Here's how the part is built. I have some questions about the finished solid (model axes, mm). A direction names the side the tool comes from. Coordinates: 2 decimals unless noted, no trailing zeros. Write each loop counter-clockwise with the first axis right and the second up, starting at its lowest first coordinate (ties: lowest second). Pieces come first, ordered by that corner, then holes.
(1) For pin 1 Ø12 at (x, y) = (18.5, -2.5) entering from -Z; pin 2 Ø12 at (y, z) = (-14.5, -13.5) entering from +X; pin 3 Ø1 at (x, y) = (92, 4) entering from +Z, each with a flat end and sliding along its axis, tell me the tip position at first contact or that it passes through.
(2) Please list where these lines run through material, in increasing order: probe 1 along X at (y, z) = (-18, -4); probe 2 along Y at (x, z) = (122, 7); probe 3 along Z at (x, y) = (74, -0.5).
(3) Which directions (+Z, -Z, +X, -X, +Y, -Y) give clear straight access to the entire face, cutting with the end or side of a thin tool? Please do faces 1 (the cylindrical face through (65.314, -14.985, 0.66)), 2 (the flat face through (-10, 0, 23)).
(4) Imagine slicing it at A-A, the plane x = 8.5. List the corners of the cut face in (y, z) for me.
Autodesk Inventor part; units mm, degrees
ref_plane "Work Plane1" through (1.525, 0, 0) normal (0, 0, 1) x (1, 0, 0)
ref_plane "YZ Plane" through (0, 0, 0) normal (1, 0, 0) x (0, 1, 0)
ref_plane "XZ Plane" through (0, 0, 0) normal (0, 1, 0) x (-1, 0, 0)
sketch "Sketch1" plane through (0, 0, 0) normal (0, 0, 1) x (1, 0, 0)
  line L0 (0, 15) -> (130, 15)
  line L1 (130, 15) -> (130, 0)
  line L2 (130, 0) -> (0, 0)
  line L3 (-26, 0) -> (156, 0)
  line L4 (0, -3) -> (0, 18)
  line L5 (0, 15) -> (0, 0)
  dimension "d2" = 30
  dimension "d59" = 130
revolve "Body" add sketch "Sketch1" angle 360 about axis through (130, 0, 0) along (-1, 0, 0)
sketch "Sketch2" plane through (0, 0, 0) normal (-1, 0, 0) x (0, 0, 1)
  line L0 (0, 26.5581) -> (23, 13.2791)
  line L1 (23, 13.2791) -> (23, -13.2791)
  line L2 (23, -13.2791) -> (0, -26.5581)
  line L3 (0, -26.5581) -> (-23, -13.2791)
  line L4 (-23, -13.2791) -> (-23, 13.2791)
  line L5 (-23, 13.2791) -> (0, 26.5581)
  line L6 (-32.2, 0) -> (32.2, 0)
  line L7 (0, 37.1814) -> (0, -37.1814)
  point P0 (0, 0)
  point P1 (0, 0)
  dimension "d11" = 46
extrude "Head" add sketch "Sketch2" along normal blind 19.75
sketch "Sketch4" plane through (0, 0, 0) normal (0, 0, 1) x (1, 0, 0)
  line L0 (-17.0942, 27.6) -> (-19.75, 23)
  line L1 (-1.1, 0) -> (-0.234, 0)
  line L2 (-23.6532, 0) -> (3.6692, 0)
  line L3 (-19.75, 27.6) -> (-17.0942, 27.6)
  line L4 (-19.75, 23) -> (-19.75, 27.6)
  line L5 (0, 33.12) -> (0, -5.52)
  dimension "d65" = 46
  dimension "d67" = 30
  dimension "d68" = 55.2
  dimension "d69" = 19.75
revolve "Chamfer1" cut sketch "Sketch4" angle 360 about axis through (-1.1, 0, 0) along (1, 0, 0)
thread "Thread"
chamfer "Chamfer2" distance 2.1471 distance2 2.1472 1 edges at (130, -15, 0) measured on face at (130, -3.9999, -1.1966)
fillet "Fillet" radius 1 1 edges at (0, -15, 0)
ref_plane "Work Plane1" through (1.525, 0, 0) normal (0, 0, 1) x (1, 0, 0)
equation "\"d2\" = GD"
equation "\"d59\" = NLG"
equation "\"d11\" = SW"
equation "\"d3\" = KOH"
equation "\"d15\" = GEL"
equation "\"d6\" = -0.5 * SPD + 0.5 * GD"
equation "\"d71\" = RR1"
equation "\"d65\" = SW"
equation "\"d67\" = ANG1"
equation "\"d68\" = 1.2 * SW"
equation "\"d69\" = KOH"
equation "\"NLG\" = 130"
equation "\"GD\" = NND"
equation "\"KOH\" = 19.75"
equation "\"GEL\" = 72"
equation "\"SW\" = 46"
equation "\"SW0\" = SW"
equation "\"SPD\" = NND - 1.2269 * PTC"
equation "\"SD\" = 0"
equation "\"ANG1\" = 30deg"
equation "\"GAL\" = 0.61345 * PTC"
equation "\"GUL\" = 0.61345 * PTC"
equation "\"RR\" = 0.1"
equation "\"RR1\" = 1"
equation "\"GD1\" = THREADDIA - 1.2269 * PTC"
equation "\"TOA\" = 30deg"
equation "\"PTC\" = 3.5"
equation "\"KOH1\" = 13.1"
equation "\"E0\" = 1.155 * SW"
properties part number "ANSI B18.2.3.5M - M30 x 3,5 x 130" material "Steel, Mild"
Recorded:
1. pin 1: stops at z = -15
1. pin 2: stops at x = 129.04
1. pin 3: stops at z = 14.59
2. probe 1: x = -19.75 to 0
2. probe 2: y = -13.27 to 13.27
2. probe 3: z = -14.99 to 14.99
3. face 1: +X
3. face 2: +Z, +X, -X, +Y, -Y
4. outline: circle Ø30 at (0, 0)
